Part model, mm, in its own coordinate system. A direction names the side the tool comes from. Round coordinates to 2 decimals unless told otherwise and drop trailing zeros. Loops run counter-clockwise (first coordinate to the right, second up) from the corner with the lowest first, then second, coordinate; pieces in that order, holes last. Notation, with made-up numbers: (71, 74.5) -> (102, 74.5) arc R17 ccw to (102, 83.5) -> close; hole circle Ø11 at (44.25, 75.5). An arc over 180 degrees is marked (long way). Answer as CSV lines item,"result".
Autodesk Inventor part; units mm, degrees
ref_plane "YZ Plane" through (0, 0, 0) normal (1, 0, 0) x (0, 1, 0)
ref_plane "XZ Plane" through (0, 0, 0) normal (0, 1, 0) x (-1, 0, 0)
ref_plane "XY Plane" through (0, 0, 0) normal (0, 0, 1) x (1, 0, 0)
sketch "スケッチ1" plane through (0, 0, 0) normal (1, 0, 0) x (0, 1, 0)
  line L0 (0, 0) -> (-9, 0)
  line L1 (-9, 0) -> (-9, 9)
  line L2 (-9, 9) -> (0, 9)
  line L3 (0, 9) -> (0, 0)
  line L4 (-1.2, 7.8) -> (-7.8, 7.8)
  line L5 (-7.8, 7.8) -> (-7.8, 1.2)
  line L6 (-7.8, 1.2) -> (-1.2, 1.2)
  line L7 (-1.2, 1.2) -> (-1.2, 7.8)
  dimension "d0" = 9
  dimension "d1" = 9
  dimension "d2" = 6.6
  dimension "d3" = 6.6
  dimension "d4" = 1.2
  dimension "d5" = 6.6
  dimension "d6" = 1.2
extrude "押し出し1" add sketch "スケッチ1" along normal blind 18
sketch "スケッチ2" plane through (0, -9, 9) normal (0, 0, 1) x (1, 0, 0)
  line L0 (0, 9) -> (0, 0)
  line L1 (0, 9) -> (18, 9)
  point P0 (4.5, 4.5)
  dimension "d9" = 4.5
  dimension "d10" = 4.5
hole "穴1" at (4.5, -4.5, 9) direction (0, 0, -1) diameter 3 end through all
sketch "スケッチ3" plane through (0, 0, 9) normal (0, 1, 0) x (1, 0, 0)
  line L0 (18, 9) -> (18, 0)
  line L1 (0, 9) -> (18, 9)
  point P0 (13.5, 4.5)
  dimension "d18" = 4.5
  dimension "d19" = 4.5
hole "穴2" at (13.5, 0, 4.5) direction (0, -1, 0) diameter 3 end through all
sketch "スケッチ4" plane through (0, -9, 0) normal (0, -1, 0) x (1, 0, 0)
  line L0 (0, 9) -> (0, 0)
  line L1 (0, 0) -> (18, 0)
  point P0 (4.5, 4.5)
  dimension "d27" = 4.5
  dimension "d28" = 4.5
hole "穴3" at (4.5, -9, 4.5) direction (0, 1, 0) diameter 6 end through all
properties part number "上下直動9x9x18" material "アルミニウム 6061"
Q1. Two-plate mould, pull along X, no slides. Class faces 1 (the face through (4.05, -5.93, 8.39)), 2 (the face through (18, -1, 5)), 3 (the face through (9, -5, 9)): pulls with the +X half, pulls with the -X half, needs draft (parallel to the pull), parting line crosses it, or undercut.
Geometry results:
face 1,"undercut"
face 2,"pulls with the +X half"
face 3,"needs draft"
Q2. Saw through at C-C, the plane x = 4.5. Write the cut outline in (y, z).
Geometry results:
outline,"(-9, 0) -> (-6, 0) -> (-6, 1.2) -> (-7.8, 1.2) -> (-7.8, 1.5) -> (-9, 1.5) -> close; (-9, 7.5) -> (-7.8, 7.5) -> (-7.8, 7.8) -> (-6, 7.8) -> (-6, 9) -> (-9, 9) -> close; (-3, 0) -> (0, 0) -> (0, 1.5) -> (-1.2, 1.5) -> (-1.2, 1.2) -> (-3, 1.2) -> close; (-3, 7.8) -> (-1.2, 7.8) -> (-1.2, 7.5) -> (0, 7.5) -> (0, 9) -> (-3, 9) -> close"
Q3. Saw through at A-A, the plane x = 13.5. Write the cut outline in (y, z).
Geometry results:
outline,"(-9, 0) -> (0, 0) -> (0, 3) -> (-1.2, 3) -> (-1.2, 1.2) -> (-7.8, 1.2) -> (-7.8, 3) -> (-9, 3) -> close; (-9, 6) -> (-7.8, 6) -> (-7.8, 7.8) -> (-1.2, 7.8) -> (-1.2, 6) -> (0, 6) -> (0, 9) -> (-9, 9) -> close"
Q4. Which spindle directions (+Z, -Z, +X, -X, +Y, -Y) get a long thin tool onto all of the face, cutting with end or side? Do faces 4 (the face through (9, -5, 1.2)), 5 (the face through (9, -9, 4)). Say none if no direction does.
Geometry results:
face 4,"+X, -X"
face 5,"+Z, -Z, +X, -X, -Y"
Q5. Drill centre lines: line 1 along X through (y, z) = (-8.2, 4.5); line 2 along Z through (x, y) = (14.5, -4.25); line 3 along Y through (x, z) = (4.5, 0.3). Where is each one in solid material? Low to high.
Geometry results:
line 1,"0 to 1.5, 7.5 to 12, 15 to 18"
line 2,"0 to 1.2, 7.8 to 9"
line 3,"-9 to -6, -3 to 0"
Q6. Saw through at B-B, the plane y = -2.75. Write the cut outline in (x, z).
Geometry results:
outline,"(0, 0) -> (18, 0) -> (18, 1.2) -> (0, 1.2) -> close; (0, 7.8) -> (18, 7.8) -> (18, 9) -> (0, 9) -> close"
Q7. Saw through at D-D, the plane z = 4.5. Write the cut outline in (x, y).
Geometry results:
outline,"(0, -9) -> (1.5, -9) -> (1.5, -7.8) -> (0, -7.8) -> close; (0, -1.2) -> (1.5, -1.2) -> (1.5, 0) -> (0, 0) -> close; (7.5, -9) -> (12, -9) -> (12, -7.8) -> (7.5, -7.8) -> close; (7.5, -1.2) -> (12, -1.2) -> (12, 0) -> (7.5, 0) -> close; (15, -9) -> (18, -9) -> (18, -7.8) -> (15, -7.8) -> close; (15, -1.2) -> (18, -1.2) -> (18, 0) -> (15, 0) -> close"
